Read the model definition and answer for the solid it produces. Units are mm, in the model's axes. A direction names the side the tool comes from. Coordinates: 2 decimals unless noted, no trailing zeros. Loops run counter-clockwise (first coordinate to the right, second up) from the corner with the lowest first, then second, coordinate; pieces in that order, holes last. Notation, with made-up numbers: (1.5, 71.5) -> (33.5, 71.5) arc R5 ccw to (33.5, 75.5) -> close; hole circle Ø9 at (-27.5, 40.25). An arc over 180 degrees is marked (long way). Answer as a JSON object with one key per item and string values. Group by question number.
Q1. For faces 1 (the flat face through (6, -12, -23.824)), 2 (the flat face through (-42, -25, 6)), determine the directions among +Z, -Z, +X, -X, +Y, -Y from which every point of the face is accessible in a straight line to the end or side of a thin tool.
Q2. Straight lines are drawn through the part: line 1 along X through (y, z) = (-21.5, -32); line 2 along Z through (x, y) = (-5, -14); line 3 along Z through (x, y) = (7.5, -21). For each, find the intervals that lie inside material, in ascending order. Write a range as [from, to].
Q3. The part is cut by section A-A on z = -34. Write down the section's boundary in (x, y).
Q4. The part is cut by section B-B on x = -141. Write down the section's boundary in (y, z).
Q5. The part is cut by section C-C on y = -17.5. State how many separate pieces and enclosed holes the cut face has, and give its area (3 significant figures).
Q6. Determine the mould class of faces 3 (the flat face through (61.937, -12, -6)), 4 (the flat face through (45, -12, 12.59)) for opening direction Z: released by +Z, released by -Z, zero draft, split by the parting line, or undercut.
Q7. Each of these flat-tipped pins is pushed along its axis until it touches: P1, Ø10, axis at x = -62.5, y = -7.5, coming from the +Z side; P2, Ø2, axis at x = -93, z = 15, coming from the +Y side; P3, Ø6.5, axis at x = -58, y = -12.5, coming from the -Z side; P4, Ø8, axis at y = -9.5, z = -40, coming from the -X side. Where does it stop, or does it pass through?
from build123d import *

# Parameters (mm, degrees)
F0_R     = 35.3591127091
F1_DEPTH = 25


with BuildPart() as f1:
    # F0 (on Front) → F1 (new body)
    with BuildSketch(Plane.XZ):
        with BuildLine():
            Line((61.9367249054, 34.8669122506), (-123.0632750946, 34.8669122506))
            Line((-123.0632750946, 34.8669122506), (-123.0632750946, 21.6819903858))
            ThreePointArc((-123.0632750946, 21.6819903858), (-116.6274794012, 9.4492653106), (-114.4056740389, -4.193410743))
            ThreePointArc((-114.4056740389, -4.193410743), (-116.6274794012, -17.8360867967), (-123.0632750946, -30.0688118719))
            Line((-123.0632750946, -30.0688118719), (-123.0632750946, -45.8291395163))
            Line((-123.0632750946, -45.8291395163), (61.9367249054, -45.8291395163))
            Line((61.9367249054, -45.8291395163), (61.9367249054, 34.8669122506))
        make_face()
        with BuildLine():
            add(Edge.make_bspline(
                [(-81.4851504642, 6.2619487625), (-83.2026240645, 6.7321619524), (-84.9001733771, 6.7321619524)],
                knots=[0, 0, 0, 1, 1, 1], degree=2))
            add(Edge.make_bspline(
                [(-84.9001733771, 6.7321619524), (-88.1836959912, 6.7321619524), (-90.8137019684, 4.7158240365)],
                knots=[0, 0, 0, 1, 1, 1], degree=2))
            add(Edge.make_bspline(
                [(-90.8137019684, 4.7158240365), (-93.4437079457, 2.6994861206), (-95.0376509623, -1.2216137001)],
                knots=[0, 0, 0, 1, 1, 1], degree=2))
            add(Edge.make_bspline(
                [(-95.0376509623, -1.2216137001), (-96.6315939788, -5.1427135208), (-96.6315939788, -9.6535722576)],
                knots=[0, 0, 0, 1, 1, 1], degree=2))
            add(Edge.make_bspline(
                [(-96.6315939788, -9.6535722576), (-96.6315939788, -13.8137635308), (-94.9260749511, -15.8301014467)],
                knots=[0, 0, 0, 1, 1, 1], degree=2))
            add(Edge.make_bspline(
                [(-94.9260749511, -15.8301014467), (-93.2205559234, -17.8464393626), (-89.4827595496, -17.8464393626)],
                knots=[0, 0, 0, 1, 1, 1], degree=2))
            add(Edge.make_bspline(
                [(-89.4827595496, -17.8464393626), (-85.8485694719, -17.8464393626), (-81.0667404223, -15.9257380277)],
                knots=[0, 0, 0, 1, 1, 1], degree=2))
            Line((-81.0667404223, -15.9257380277), (-81.0667404223, -22.4051163899))
            add(Edge.make_bspline(
                [(-81.0667404223, -22.4051163899), (-86.0159334887, -24.3258177248), (-91.0288842757, -24.3258177248)],
                knots=[0, 0, 0, 1, 1, 1], degree=2))
            add(Edge.make_bspline(
                [(-91.0288842757, -24.3258177248), (-97.3488683362, -24.3258177248), (-100.8635126877, -20.5999759237)],
                knots=[0, 0, 0, 1, 1, 1], degree=2))
            add(Edge.make_bspline(
                [(-100.8635126877, -20.5999759237), (-104.3781570392, -16.8741341225), (-104.3781570392, -10.0520580117)],
                knots=[0, 0, 0, 1, 1, 1], degree=2))
            add(Edge.make_bspline(
                [(-104.3781570392, -10.0520580117), (-104.3781570392, -3.524861359), (-101.7879996373, 1.9662723329)],
                knots=[0, 0, 0, 1, 1, 1], degree=2))
            add(Edge.make_bspline(
                [(-101.7879996373, 1.9662723329), (-99.1978422354, 7.4574060249), (-94.8623172304, 10.3105640245)],
                knots=[0, 0, 0, 1, 1, 1], degree=2))
            add(Edge.make_bspline(
                [(-94.8623172304, 10.3105640245), (-90.5267922255, 13.1637220241), (-84.9001733771, 13.1637220241)],
                knots=[0, 0, 0, 1, 1, 1], degree=2))
            add(Edge.make_bspline(
                [(-84.9001733771, 13.1637220241), (-81.7840147798, 13.1637220241), (-79.3691911097, 12.6018571108)],
                knots=[0, 0, 0, 1, 1, 1], degree=2))
            add(Edge.make_bspline(
                [(-79.3691911097, 12.6018571108), (-76.9543674396, 12.0399921975), (-74.188876306, 10.549655477)],
                knots=[0, 0, 0, 1, 1, 1], degree=2))
            Line((-74.188876306, 10.549655477), (-77.1297011715, 4.3173382823))
            add(Edge.make_bspline(
                [(-77.1297011715, 4.3173382823), (-79.7676768638, 5.7917355726), (-81.4851504642, 6.2619487625)],
                knots=[0, 0, 0, 1, 1, 1], degree=2))
        make_face(mode=Mode.SUBTRACT)
        Polygon((-54.5594680573, -23.8237256746), (-74.9061506634, -23.8237256746), (-67.2153756086, 12.5899025382), (-59.5883582745, 12.5899025382), (-65.9641303406, -17.4479536085), (-53.2125862083, -17.4479536085), align=None, mode=Mode.SUBTRACT)
        Polygon((-28.2354991392, -23.8237256746), (-28.8332277704, -15.1526756647), (-40.6124666626, -15.1526756647), (-44.892203662, -23.8237256746), (-52.8619187447, -23.8237256746), (-33.7903905518, 12.7413271247), (-24.4977027654, 12.7413271247), (-20.8396035425, -23.8237256746), align=None, mode=Mode.SUBTRACT)
        with BuildLine():
            Line((-2.9236840366, -9.8528151347), (-5.8884180473, -9.8528151347))
            Line((-5.8884180473, -9.8528151347), (-8.8531520581, -23.8237256746))
            Line((-8.8531520581, -23.8237256746), (-16.4482905319, -23.8237256746))
            Line((-16.4482905319, -23.8237256746), (-8.7575154771, 12.5899025382))
            Line((-8.7575154771, 12.5899025382), (0.1845048457, 12.5899025382))
            add(Edge.make_bspline(
                [(0.1845048457, 12.5899025382), (6.0900637219, 12.5899025382), (9.0547977327, 10.0475634268)],
                knots=[0, 0, 0, 1, 1, 1], degree=2))
            add(Edge.make_bspline(
                [(9.0547977327, 10.0475634268), (12.0195317435, 7.5052243154), (12.0195317435, 2.6038495396)],
                knots=[0, 0, 0, 1, 1, 1], degree=2))
            add(Edge.make_bspline(
                [(12.0195317435, 2.6038495396), (12.0195317435, -1.3331897113), (9.9513906795, -4.1584537081)],
                knots=[0, 0, 0, 1, 1, 1], degree=2))
            add(Edge.make_bspline(
                [(9.9513906795, -4.1584537081), (7.8832496155, -6.9837177049), (3.9940286552, -8.3545086991)],
                knots=[0, 0, 0, 1, 1, 1], degree=2))
            Line((3.9940286552, -8.3545086991), (10.4973161627, -23.8237256746))
            Line((10.4973161627, -23.8237256746), (2.2247519068, -23.8237256746))
            Line((2.2247519068, -23.8237256746), (-2.9236840366, -9.8528151347))
        make_face(mode=Mode.SUBTRACT)
        Polygon((34.4542797012, -4.8478340628), (41.7067204265, -23.8237256746), (33.2827315841, -23.8237256746), (28.0306893446, -9.0797527717), (24.9145307472, -10.8251203748), (22.2048276191, -23.8237256746), (14.6096891453, -23.8237256746), (22.3004642001, 12.5899025382), (29.9274815343, 12.5899025382), (26.14186687, -4.8956523532), (30.0709364057, 0.2129350148), (40.2562322814, 12.5899025382), (49.2540406098, 12.5899025382), align=None, mode=Mode.SUBTRACT)
        with BuildLine():
            ThreePointArc((-114.4056740389, -4.193410743), (-116.6274794012, 9.4492653106), (-123.0632750946, 21.6819903858))
            ThreePointArc((-123.0632750946, 21.6819903858), (-200.3983681841, -4.193410743), (-123.0632750946, -30.0688118719))
            ThreePointArc((-123.0632750946, -30.0688118719), (-116.6274794012, -17.8360867967), (-114.4056740389, -4.193410743))
        make_face()
        with Locations((-157.4020211115, -4.193410743)):
            Circle(F0_R, mode=Mode.SUBTRACT)
    extrude(amount=F1_DEPTH)


solid = f1.part
Final values:
{
 "1": {"face 1": "+Y, -Y", "face 2": "+Z, -Z, +X, -X, -Y"},
 "2": {"line 1": "x = [-190.2, -179.24], [-135.56, -124.61], [-123.06, 61.94]", "line 2": "z = [-45.83, -9.85], [12.59, 34.87]", "line 3": "z = [-45.83, -23.82], [-16.69, -6.57], [11.1, 34.87]"},
 "3": {"outline": "(-188.39, -25) -> (-176.42, -25) -> (-176.42, 0) -> (-188.39, 0) -> close; (-138.38, -25) -> (-126.41, -25) -> (-126.41, 0) -> (-138.38, 0) -> close; (-123.06, -25) -> (61.94, -25) -> (61.94, 0) -> (-123.06, 0) -> close"},
 "4": {"outline": "(-25, -43.94) -> (0, -43.94) -> (0, -35.52) -> (-25, -35.52) -> close; (-25, 27.13) -> (0, 27.13) -> (0, 35.55) -> (-25, 35.55) -> close"},
 "5": {"separate pieces": "1", "enclosed holes": "6", "area": "13,800 mm2"},
 "6": {"face 3": "zero draft", "face 4": "undercut"},
 "7": {"P1": "stops at z = 34.87", "P2": "stops at y = 0", "P3": "stops at z = -45.83", "P4": "stops at x = -186.33"}
}
